Autodesk Inventor part; units mm, degrees
ref_plane "YZ Plane" through (0, 0, 0) normal (1, 0, 0) x (0, 1, 0)
ref_plane "XZ Plane" through (0, 0, 0) normal (0, 1, 0) x (-1, 0, 0)
ref_plane "XY Plane" through (0, 0, 0) normal (0, 0, 1) x (1, 0, 0)
sketch "Sketch1" plane through (0, 0, 0) normal (0, 0, 1) x (1, 0, 0)
  line L0 (-31.5, 17.5) -> (31.5, 17.5)
  line L1 (31.5, 17.5) -> (31.5, -17.5)
  line L2 (31.5, -17.5) -> (-31.5, -17.5)
  line L3 (-31.5, -17.5) -> (-31.5, 17.5)
  line L4 (-31.5, 17.5) -> (31.5, -17.5) construction
  line L5 (31.5, 17.5) -> (-31.5, -17.5) construction
  circle A0 centre (13.6, 0.2) radius 4
  circle A1 centre (-17.45, 3.08) radius 2.5
  circle A2 centre (-17.45, -3.3) radius 2.5
  point P0 (0, 0)
  dimension "d0" = 63
  dimension "d1" = 35
  dimension "d2" = 8
  dimension "d3" = 17.9
  dimension "d4" = 17.7
  dimension "d5" = 5
  dimension "d6" = 5
  dimension "d7" = 14.2
  dimension "d8" = 48.95
  dimension "d9" = 48.95
  dimension "d10" = 20.58
extrude "Extrusion1" add sketch "Sketch1" along normal blind 3
sketch "Sketch2" plane through (0, 0, 3) normal (0, 0, 1) x (1, 0, 0)
  circle A0 centre (25.16, 0) radius 2
  line L0 (31.5, -17.5) -> (31.5, 17.5)
  line L1 (-31.5, -17.5) -> (31.5, -17.5)
  circle A1 centre (-25.16, 0) radius 2
  line L2 (-31.5, 17.5) -> (-31.5, -17.5)
  point P0 (0, 0)
  dimension "d13" = 6.34
  dimension "d14" = 17.5
  dimension "d15" = 4
  dimension "d16" = 4
  dimension "d17" = 6.34
  dimension "d18" = 17.5
extrude "Extrusion2" cut sketch "Sketch2" against normal blind 3
equation "\"d9\" = d8"
equation "\"d17\" = d13"
equation "\"d18\" = d14"
properties part number "EndCapCutout"
Build history of the part. All positions in model axes, mm. Round coordinates to 2 decimals unless told otherwise and drop trailing zeros. Loops run counter-clockwise (first coordinate to the right, second up) from the corner with the lowest first, then second, coordinate; pieces in that order, holes last. Notation, with made-up numbers: (62, 75) -> (114, 75) arc R17 ccw to (114, 99) -> close; hole circle Ø11 at (-3.5, 50.25). An arc over 180 degrees is marked (long way). One line per item, written item: value. Start each with the question number.
Q1. Cut at C-C on x = -17.45. List the corners of the cut face in (y, z).
Q2. Drop a flat-ended pin along its axis: pin 1 Ø4 at (x, y) = (18.5, -2.5) entering from -Z. Give the stop position or say it passes through.
Q3. Probe line 1 along Y through (x, z) = (-17.45, 1.35); line 2 along X through (y, z) = (3, 1); line 3 along Y through (x, z) = (-25.16, 1.25). List the from-to ranges inside material, lowest first.
Q4. Two-plate mould, pull along X, no slides. Class faces 1 (the face through (-31.5, 0, 1)), 2 (the face through (0, 17.5, 1)), 3 (the face through (-19.434, -1.779, 1.479)): released by +X, released by -X, zero draft, split by the parting line, or undercut.
Q5. Cut at A-A on z = 2.45. List the corners of the cut face in (x, y).
Q6. Cut at B-B on x = -25.16. List the corners of the cut face in (y, z), plus the area to 3 significant figures.
Q7. Cut at D-D on x = 13.6. List the corners of the cut face in (y, z).
Computed:
1. outline: (-17.5, 0) -> (-5.8, 0) -> (-5.8, 3) -> (-17.5, 3) -> close; (-0.8, 0) -> (0.58, 0) -> (0.58, 3) -> (-0.8, 3) -> close; (5.58, 0) -> (17.5, 0) -> (17.5, 3) -> (5.58, 3) -> close
2. pin 1: z = 0
3. line 1: -17.5 to -5.8, -0.8 to 0.58, 5.58 to 17.5
3. line 2: -31.5 to -19.95, -14.95 to 10.74, 16.46 to 31.5
3. line 3: -17.5 to -2, 2 to 17.5
4. face 1: released by -X
4. face 2: zero draft
4. face 3: undercut
5. outline: (-31.5, -17.5) -> (31.5, -17.5) -> (31.5, 17.5) -> (-31.5, 17.5) -> close; hole circle Ø4 at (-25.16, 0); hole circle Ø5 at (-17.45, -3.3); hole circle Ø5 at (-17.45, 3.08); hole circle Ø8 at (13.6, 0.2); hole circle Ø4 at (25.16, 0)
6. outline: (-17.5, 0) -> (-2, 0) -> (-2, 3) -> (-17.5, 3) -> close; (2, 0) -> (17.5, 0) -> (17.5, 3) -> (2, 3) -> close
6. area: 93.0 mm²
7. outline: (-17.5, 0) -> (-3.8, 0) -> (-3.8, 3) -> (-17.5, 3) -> close; (4.2, 0) -> (17.5, 0) -> (17.5, 3) -> (4.2, 3) -> close
